The figure shows three views and two pictorial views of one solid part (mm, origin at its lowest corner). Answer the questions. Coordinates: 2 decimals unless noted, no trailing zeros. Write each loop counter-clockwise with the first axis right and the second up, starting at its lowest first coordinate (ties: lowest second). Pieces come first, ordered by that corner, then holes. Notation, with made-up numbers: M 24,52 L 64,52 A21 cw 64,72 Z; hole C 24.5,-28 d7. An arc over 180 degrees is marked long. Write item = value, one per line. Start each with the question number.
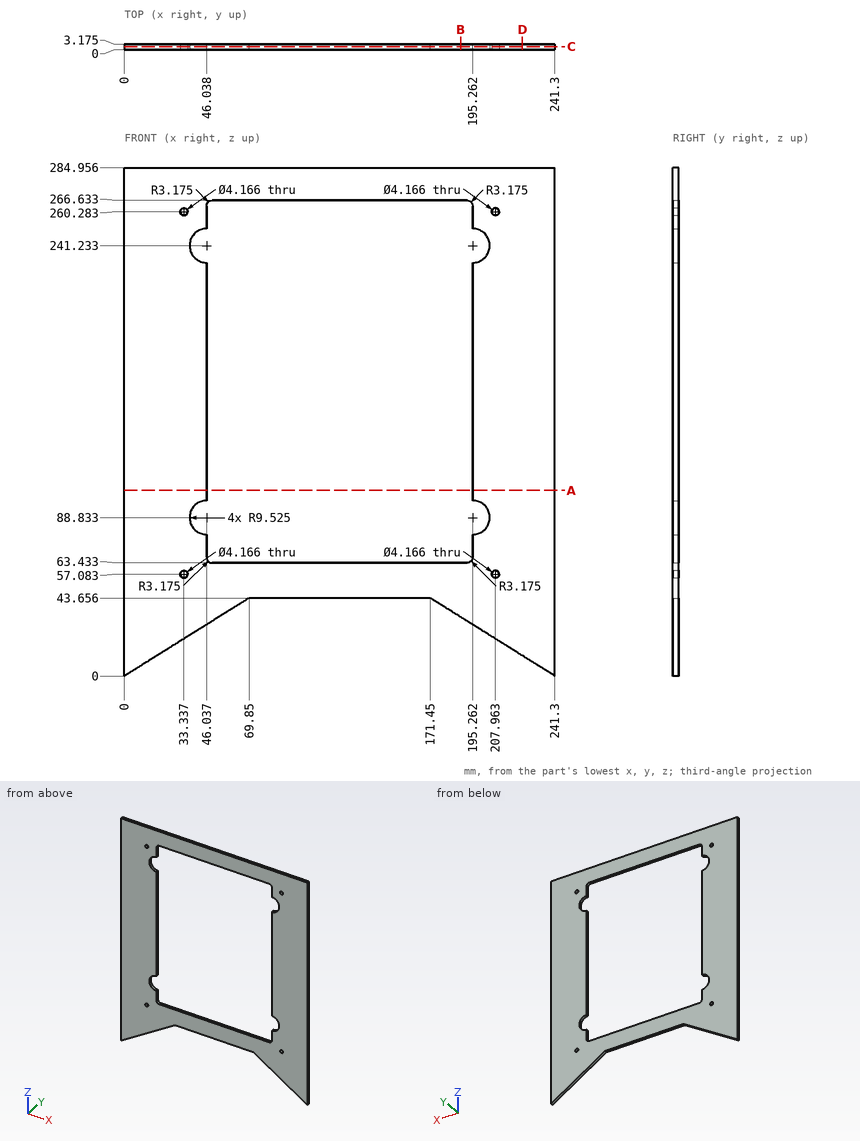
1. Each of these flat-tipped pins is pushed along its axis until it touches: pin 1 (1 mm diameter, centred on x = 100.5, y = 1.5, fed in from -Z); pin 2 (1 mm diameter, centred on x = 30, y = 2, fed in from -Z). Where does it stop, or does it pass through?
2. The part is cut by section A-A, the plane z = 104. Write down the section's boundary in (x, y) (1 decimal).
3. The part is cut by section C-C, the plane y = 1.75. Count the separate pieces of the cut face and the enclosed holes in it, and give its area (3 significant figures).
4. The part is cut by section D-D, the plane x = 223. Write down the section's boundary in (y, z) (1 decimal).
5. Straight lines are drawn through the part: L1, parallel to X at y = 1.75, z = 184; L2, parallel to Z at x = 132, y = 0.2; L3, parallel to Z at x = 200.5, y = 0.3 (1 decimal). For each, find the intervals that lie inside material, in ascending order. Write a range as [from, to].
6. The part is cut by section B-B, the plane x = 188.5. Write down the section's boundary in (y, z) (1 decimal), and give its area (3 significant figures).
Solution:
q1.pin_1 = 43.66
q1.pin_2 = 18.44
q2.outline = M 0,0 L 46,0 L 46,3.2 L 0,3.2 Z; M 195.3,0 L 241.3,0 L 241.3,3.2 L 195.3,3.2 Z
q3.separate_pieces = 1
q3.enclosed_holes = 5
q3.area = 30,300 mm^2
q4.outline = M 0,11.4 L 3.2,11.4 L 3.2,285 L 0,285 Z
q5.L1 = [0, 46.04], [195.26, 241.3]
q5.L2 = [43.66, 63.43], [266.63, 284.96]
q5.L3 = [25.5, 80.9], [96.8, 233.3], [249.2, 285]
q6.outline = M 0,33 L 3.2,33 L 3.2,63.4 L 0,63.4 Z; M 0,266.6 L 3.2,266.6 L 3.2,285 L 0,285 Z
q6.area = 155 mm^2
